```python
from build123d import *

# Parameters (mm, degrees)
HANDBRAKE_TOP_SUPPORT_EXTRUDE_DEPTH = 191.5
HANDBRAKE_TOP_SUPPORT_CUT_REACH     = 195.529


with BuildPart() as part:
    # Sketch1<8> → handbrake top support extrude (new body)
    with BuildSketch(Plane(origin=(0, 0, 0), x_dir=(0, 0, -1), z_dir=(1, 0, 0))):
        with BuildLine():
            Line((10.5, 12.5), (-10.5, 12.5))
            ThreePointArc((-10.5, 12.5), (-11.914213562, 11.914213562), (-12.5, 10.5))
            Line((-12.5, 10.5), (-12.5, -10.5))
            ThreePointArc((-12.5, -10.5), (-11.914213562, -11.914213562), (-10.5, -12.5))
            Line((-10.5, -12.5), (10.5, -12.5))
            ThreePointArc((10.5, -12.5), (11.914213562, -11.914213562), (12.5, -10.5))
            Line((12.5, -10.5), (12.5, 10.5))
            ThreePointArc((12.5, 10.5), (11.914213562, 11.914213562), (10.5, 12.5))
        make_face()
        with BuildLine():
            Line((-9.5, 10.5), (9.5, 10.5))
            ThreePointArc((9.5, 10.5), (10.207106781, 10.207106781), (10.5, 9.5))
            Line((10.5, 9.5), (10.5, -9.5))
            ThreePointArc((10.5, -9.5), (10.207106781, -10.207106781), (9.5, -10.5))
            Line((9.5, -10.5), (-9.5, -10.5))
            ThreePointArc((-9.5, -10.5), (-10.207106781, -10.207106781), (-10.5, -9.5))
            Line((-10.5, -9.5), (-10.5, 9.5))
            ThreePointArc((-10.5, 9.5), (-10.207106781, 10.207106781), (-9.5, 10.5))
        make_face(mode=Mode.SUBTRACT)
    extrude(amount=HANDBRAKE_TOP_SUPPORT_EXTRUDE_DEPTH)

    # Sketch7 → handbrake top support cut (cut, up to next)
    with BuildSketch(Plane.XY.offset(12.5), mode=Mode.PRIVATE) as handbrake_top_support_cut_sk1:
        Polygon((0, 12.5), (0, -12.5), (15.92675652, 12.5), align=None)
    handbrake_top_support_cut_tool1 = extrude(handbrake_top_support_cut_sk1.sketch, amount=-HANDBRAKE_TOP_SUPPORT_CUT_REACH, mode=Mode.PRIVATE) & part.part
    # Sketch7 → handbrake top support cut (cut, up to next)
    with BuildSketch(Plane.XY.offset(12.5), mode=Mode.PRIVATE) as handbrake_top_support_cut_sk2:
        Polygon((191.5, -12.5), (175.57324348, 12.5), (191.5, 12.5), align=None)
    handbrake_top_support_cut_tool2 = extrude(handbrake_top_support_cut_sk2.sketch, amount=-HANDBRAKE_TOP_SUPPORT_CUT_REACH, mode=Mode.PRIVATE) & part.part
    add(handbrake_top_support_cut_tool1.solids().sort_by_distance((5.308919, 4.166667, 12.5))[0], mode=Mode.SUBTRACT)
    add(handbrake_top_support_cut_tool2.solids().sort_by_distance((186.191081, 4.166667, 12.5))[0], mode=Mode.SUBTRACT)


solid = part.part
```
Could you check a few things on this model? Use its own coordinates, in mm. A direction names the side the tool comes from. Coordinates: 2 decimals unless noted, no trailing zeros. Loops run counter-clockwise (first coordinate to the right, second up) from the corner with the lowest first, then second, coordinate; pieces in that order, holes last. Notation, with made-up numbers: M 60.5,-15 L 97.5,-15 A25 cw 97.5,20 Z; hole C 28.25,41.25 d9. An arc over 180 degrees is marked long. Put each result on its own line as item: value. Start each with the question number.
(1) I need wall thicknesses on line 1 (Y direction, x = 168, z = 8.25); line 2 (Z direction, x = 56, y = 10.25). Which ranges of each line are inside material? Lowest first, please. Write a range as from..to.
(2) Suppose I cut it at B-B on x = 110. Please give me the cut outline in (y, z).
(3) Suppose I cut it at A-A on z = -6.5. Please give me the cut outline in (x, y), then the cut area to 3 significant figures.
(4) Suppose I cut it at C-C on y = -7.25. Please give me the cut outline in (x, z), then the cut area to 3 significant figures.
(5) Thinking about a two-plate mould opening in Y: for faces 1 (the face through (94, 0, -12.5)), 2 (the face through (94, -12.5, 0)), 3 (the face through (94, 0, -10.5)), which applies, pulls with the +Y half, pulls with the -Y half, needs draft (parallel to the pull), parting line crosses it, or undercut?
(6) For faces 4 (the face through (95, 10.5, 0)), 5 (the face through (94, 0, 12.5)), which set-ups out of +Z, -Z, +X, -X, +Y, -Y let a thin tool reach every point of the face, with its end or its side?
Solutions:
1. line 1: y = -12.5..-10.5, 10.5..12.5
1. line 2: z = -12.5..-10.16, 10.16..12.5
2. outline: M -12.5,-10.5 A2 ccw -10.5,-12.5 L 10.5,-12.5 A2 ccw 12.5,-10.5 L 12.5,10.5 A2 ccw 10.5,12.5 L -10.5,12.5 A2 ccw -12.5,10.5 Z; hole M -10.5,-9.5 A1 ccw -9.5,-10.5 L 9.5,-10.5 A1 ccw 10.5,-9.5 L 10.5,9.5 A1 ccw 9.5,10.5 L -9.5,10.5 A1 ccw -10.5,9.5 Z
3. outline: M 0,-12.5 L 191.5,-12.5 L 190.23,-10.5 L 1.27,-10.5 Z; M 14.65,10.5 L 176.85,10.5 L 175.57,12.5 L 15.93,12.5 Z
3. area: 702 mm2
4. outline: M 3.34,-12.5 L 188.16,-12.5 L 188.16,-10.5 L 3.34,-10.5 Z; M 3.34,10.5 L 188.16,10.5 L 188.16,12.5 L 3.34,12.5 Z
4. area: 739 mm2
5. face 1: needs draft
5. face 2: pulls with the -Y half
5. face 3: undercut
6. face 4: +X, -X
6. face 5: +Z, +X, -X, +Y, -Y
